Here's how the part is built. I have some questions about the finished solid (model axes, mm). A direction names the side the tool comes from. Round coordinates to 2 decimals unless told otherwise and drop trailing zeros. Write each loop counter-clockwise with the first axis right and the second up, starting at its lowest first coordinate (ties: lowest second). Pieces come first, ordered by that corner, then holes. Notation, with made-up numbers: (-6, 87) - (22, 87) arc R19 cw to (22, 115) - close; hole circle Ø1 at (39, 9.25). An arc over 180 degrees is marked (long way). One line per item, written item: value. Start each with the question number.
Item 1: For P1, Ø1, axis at y = 12, z = 9, coming from the -X side; P2, Ø2, axis at x = -16.5, y = -16, coming from the +Z side; P3, Ø5.5, axis at x = -15.348, y = -19.431, coming from the -Z side, each with a flat end and sliding along its axis, tell me the tip position at first contact or that it passes through.
Item 2: Imagine slicing it at C-C, the plane y = -7. Please give me the cut outline in (x, z), then the cut area to 3 significant figures.
Item 3: Thinking about a two-plate mould opening in X: for faces 1 (the face through (-21, 0, -1.1)), 2 (the face through (-8.65, 34.58, 22.34)), 3 (the face through (-17, 32, 42)), which applies, released by +X, released by -X, zero draft, split by the parting line, or undercut?
Item 4: If I drill on line 1 (Y direction, x = -20.5, z = 6); line 2 (Y direction, x = -17, z = 32.5); line 3 (X direction, y = -31.5, z = 11), over which ranges is the centre line in solid material (lowest first)?
Item 5: For faces 4 (the face through (-16.163, -30.567, 19.35)), 5 (the face through (-17.698, -32, 41)), 6 (the face through (-8.62, -33.2, -3.1)), 7 (the face through (-15, 28.35, 23)), 8 (the face through (-8.62, 0.45, -4.4)), which set-ups out of +Z, -Z, +X, -X, +Y, -Y let a thin tool reach every point of the face, with its end or its side?
Item 6: Imagine slicing it at A-A, the plane z = 14. Please give me the cut outline in (x, y), then the cut area to 3 significant figures.
Item 7: Imagine slicing it at B-B, the plane x = -11. Please give me the cut outline in (y, z), then the cut area to 3 significant figures.
```python
from build123d import *

# Parameters (mm, degrees)
PAD039_DEPTH         = 11.65
POCKET045_DEPTH      = 2.101
PAD_DEPTH            = 2
SKETCH117_W          = 9.65
SKETCH117_H          = 4.8
PAD041_DEPTH         = 46
SKETCH120_R          = 1.75
POCKET048_DEPTH      = 46.001
SKETCH115_R          = 1.75
POCKET046_DEPTH      = 5.001
SKETCH116_R          = 3
POCKET047_DEPTH      = 2.951
SKETCH118_W          = 5.65
SKETCH118_H          = 2.75
POCKET049_DEPTH      = 35.151
POCKET049_DEPTH_BACK = 35.151
FILLET_R             = 2


with BuildPart() as part:
    # Sketch119 → Pad039 (new body)
    with BuildSketch(Plane.YZ.offset(-21.698)):
        with BuildLine():
            ThreePointArc((-33.15, 1), (-32.857107, 0.292893), (-32.15, 0))
            Line((-32.15, 0), (32.15, 0))
            ThreePointArc((32.15, 0), (32.857107, 0.292893), (33.15, 1))
            Line((33.15, 46), (33.15, 1))
            Line((33.15, 46), (35.15, 46))
            Line((35.15, 46), (35.15, -2))
            Line((35.15, -2), (32.15, -5))
            Line((32.15, -5), (-32.15, -5))
            Line((-32.15, -5), (-35.15, -2))
            Line((-35.15, -2), (-35.15, 46))
            Line((-35.15, 46), (-33.15, 46))
            Line((-33.15, 46), (-33.15, 1))
        make_face()
    extrude(amount=PAD039_DEPTH)

    # Sketch114 → Pocket045 (cut, through all)
    with BuildSketch(Plane.YZ.offset(-19.598)):
        with BuildLine():
            Line((-34.25, 46), (-34.25, 1))
            ThreePointArc((-34.25, 1), (-33.634924, -0.484924), (-32.15, -1.1))
            Line((-32.15, -1.1), (32.15, -1.1))
            ThreePointArc((32.15, -1.1), (33.634924, -0.484924), (34.25, 1))
            Line((34.25, 1), (34.25, 46))
            Line((34.25, 46), (33.15, 46))
            Line((33.15, 46), (33.15, 1))
            ThreePointArc((32.15, 0), (32.857107, 0.292893), (33.15, 1))
            Line((-32.15, 0), (32.15, 0))
            ThreePointArc((-33.15, 1), (-32.857107, 0.292893), (-32.15, 0))
            Line((-33.15, 46), (-33.15, 1))
            Line((-34.25, 46), (-33.15, 46))
        make_face()
    extrude(amount=-POCKET045_DEPTH, mode=Mode.SUBTRACT)

    # Sketch123 → Pad (join)
    with BuildSketch(Plane.YZ.offset(-10.048)):
        Polygon((-35.15, 46), (-35.15, -2), (-32.15, -5), (32.15, -5), (35.15, -2), (35.15, 46), align=None)
    extrude(amount=PAD_DEPTH)

    # Sketch117 → Pad041 (join)
    with BuildSketch(Plane.XY):
        with Locations((-14.873, 30.75)):
            Rectangle(SKETCH117_W, SKETCH117_H)
        with Locations((-14.873, -30.75)):
            Rectangle(SKETCH117_W, SKETCH117_H)
    extrude(amount=PAD041_DEPTH)

    # Sketch120 → Pocket048 (cut, through all)
    with BuildSketch(Plane.XY):
        with Locations((-14.873, 31.75)):
            Circle(SKETCH120_R)
        with Locations((-14.873, -31.75)):
            Circle(SKETCH120_R)
    extrude(amount=POCKET048_DEPTH, mode=Mode.SUBTRACT)

    # Sketch115 → Pocket046 (cut, through all)
    with BuildSketch(Plane.XY):
        with Locations((-15.348, 15.621)):
            Circle(SKETCH115_R)
        with Locations((-15.348, -19.431)):
            Circle(SKETCH115_R)
    extrude(amount=-POCKET046_DEPTH, mode=Mode.SUBTRACT)

    # Sketch116 → Pocket047 (cut, through all)
    with BuildSketch(Plane.XY.offset(-2.05)):
        with Locations((-15.348, 15.621)):
            Circle(SKETCH116_R)
        with Locations((-15.348, -19.431)):
            Circle(SKETCH116_R)
    extrude(amount=-POCKET047_DEPTH, mode=Mode.SUBTRACT)

    # Sketch118 → Pocket049 (cut, two sides)
    with BuildSketch(Plane.XZ) as pocket049_sk:
        with Locations((-14.873, 40.625)):
            Rectangle(SKETCH118_W, SKETCH118_H)
    extrude(amount=-POCKET049_DEPTH, mode=Mode.SUBTRACT)
    extrude(pocket049_sk.sketch, amount=POCKET049_DEPTH_BACK, mode=Mode.SUBTRACT)

    # Fillet
    fillet_edges = [part.edges().sort_by_distance(p)[0] for p in [
        (-8.048, -35.15, 22),
        (-8.048, -33.65, -3.5),
        (-8.048, 0, -5),
        (-8.048, 33.65, -3.5),
        (-8.048, 35.15, 22),
    ]]
    fillet(fillet_edges, radius=FILLET_R)


solid = part.part
```
Values follow:
1. P1: stops at x = -10.05
1. P2: stops at z = 0
1. P3: stops at z = -2.05
2. outline: (-21.7, -5) - (-10.05, -5) arc R2 ccw to (-8.05, -3) - (-8.05, 46) - (-10.05, 46) - (-10.05, 0) - (-19.6, 0) - (-19.6, -1.1) - (-21.7, -1.1) - close
2. area: 157 mm^2
3. face 1: zero draft
3. face 2: released by +X
3. face 3: undercut
4. line 1: y = -35.15 to -34.25, 34.25 to 35.15
4. line 2: y = -35.15 to -28.35, 28.35 to 35.15
4. line 3: x = -19.7 to -16.61, -13.14 to -8.05
5. face 4: +Z
5. face 5: +Y, -Y
5. face 6: -Z, +X, -Y
5. face 7: +Z, -X
5. face 8: -Z, +X, +Y, -Y
6. outline: (-21.7, -35.15) - (-10.05, -35.15) arc R2 ccw to (-8.05, -33.15) - (-8.05, 33.15) arc R2 ccw to (-10.05, 35.15) - (-21.7, 35.15) - (-21.7, 34.25) - (-19.6, 34.25) - (-19.6, 33.15) - (-19.7, 33.15) - (-19.7, 28.35) - (-10.05, 28.35) - (-10.05, -28.35) - (-19.7, -28.35) - (-19.7, -33.15) - (-19.6, -33.15) - (-19.6, -34.25) - (-21.7, -34.25) - close; hole circle Ø3.5 at (-14.87, -31.75); hole circle Ø3.5 at (-14.87, 31.75)
6. area: 254 mm^2
7. outline: (-35.15, -2) - (-32.15, -5) - (32.15, -5) - (35.15, -2) - (35.15, 46) - (28.35, 46) - (28.35, 0) - (-28.35, 0) - (-28.35, 46) - (-35.15, 46) - close
7. area: 968 mm^2
